Design review of the part built by this model. Coordinates are the model's own, in mm. Coordinates: 2 decimals unless noted, no trailing zeros. Loops run counter-clockwise (first coordinate to the right, second up) from the corner with the lowest first, then second, coordinate; pieces in that order, holes last. Notation, with made-up numbers: M 88,12 L 100,12 A17 cw 100,24 Z; hole C 52.5,3.25 d4. An arc over 180 degrees is marked long. Answer as a JSON object with one key per item and string values. Group by question number.
1. To check wall thickness, follow probe 1 along Z at (x, y) = (76, 8.25); probe 2 along Z at (x, y) = (161, 16.25); probe 3 along Y at (x, z) = (13, -10). State the ranges of each line that lie inside material, in increasing order.
2. Consider section B-B (z = -13). State the section outline as (x, y) points (1 decimal), then the cut area to 3 significant figures.
3. Consider section C-C (x = 68). State the section outline as (y, z) points, then the cut area to 3 significant figures.
4. Consider section A-A (y = 3.75). State the section outline as (x, z) points (3 decimals), then the cut area to 3 significant figures.
5. Insertion check: pin 1 (1 mm diameter, centred on x = 39.5, z = -29.5, fed in from -Y); pin 2 (1 mm diameter, centred on x = 34, y = 17, fed in from -Z); pin 3 (11.5 mm diameter, centred on y = 6, z = -10, fed in from -X). Each pin has a flat end and moves straight along its axis. Give the tip position at first contact, or say it passes through.
6. Consider section D-D (y = 13). State the section outline as (x, z) points.
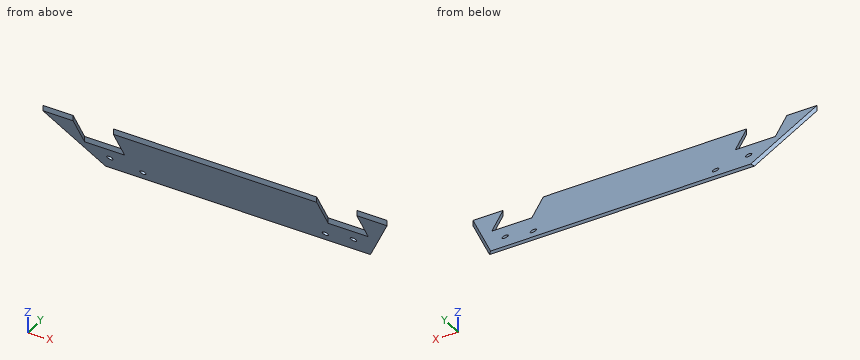
Autodesk Inventor part; units mm, degrees
ref_plane "YZ Plane" through (0, 0, 0) normal (1, 0, 0) x (0, 1, 0)
ref_plane "XZ Plane" through (0, 0, 0) normal (0, 1, 0) x (-1, 0, 0)
ref_plane "XY Plane" through (0, 0, 0) normal (0, 0, 1) x (1, 0, 0)
sketch "Szkic1" plane through (0, 0, 0) normal (1, 0, 0) x (0, 1, 0)
  line L0 (0.433, -0.75) -> (22.433, -38.8551)
  line L1 (22.433, -38.8551) -> (21.134, -39.6051)
  line L2 (21.134, -39.6051) -> (0.433, -3.75)
  line L3 (0.433, -3.75) -> (0.433, -0.75)
  line L4 (21.134, -39.6051) -> (21.134, -39.6051)
  dimension "d0" = 1.5
  dimension "d1" = 22
  dimension "d2" = 30
extrude "Wyciągnięcie proste1" add sketch "Szkic1" along normal blind 180.175
sketch "Szkic2" plane through (180.175, 22.433, 0) normal (0, 0, -1) x (-1, 0, 0)
  line L0 (143.375, -22) -> (164.375, -22)
  line L1 (164.375, -22) -> (164.375, -11.7)
  line L2 (164.375, -11.7) -> (143.375, -11.7)
  line L3 (143.375, -11.7) -> (143.375, -22)
  line L4 (180.175, -22) -> (0, -22) construction
  line L5 (180.175, -22) -> (180.175, 0) construction
  line L6 (180.175, -22) -> (180.175, 0)
  line L7 (180.175, 0) -> (0, 0) construction
  line L8 (158.175, 0) -> (180.175, -22)
  line L9 (90.0875, -22) -> (90.0875, 0) construction
  line L10 (180.175, 0) -> (158.175, 0)
  line L11 (36.8, -22) -> (15.8, -22)
  line L12 (15.8, -22) -> (15.8, -11.7)
  line L13 (15.8, -11.7) -> (36.8, -11.7)
  line L14 (36.8, -11.7) -> (36.8, -22)
  line L15 (0, -22) -> (0, 0) construction
  line L16 (0, -22) -> (0, 0)
  line L17 (22, 0) -> (0, -22)
  line L18 (0, 0) -> (22, 0)
  dimension "d9" = 21
  dimension "d10" = 10.3
  dimension "d33" = 15.8
  dimension "d34" = 45
extrude "Wyciągnięcie proste2" cut sketch "Szkic2" along normal through all
sketch "Szkic3" plane through (22, 22, -38.1051) normal (0, 0.866, 0.5) x (1, 0, 0)
  line L0 (-2, -0.5359) -> (138.175, -0.5359) construction
  line L1 (-2, -0.5359) -> (4.3275, -0.5359) construction
  line L2 (4.3275, -0.5359) -> (4.3275, -10.5359) construction
  line L3 (-2, -0.5359) -> (20.3275, -0.5359) construction
  line L4 (20.3275, -0.5359) -> (20.3275, -6.1359) construction
  line L5 (0, 0.4641) -> (136.175, 0.4641) construction
  line L6 (68.0875, 0.4641) -> (68.0854, -43.134) construction
  line L7 (-22, -43.134) -> (158.175, -43.134) construction
  circle A0 centre (20.3275, -6.1359) radius 1.6
  circle A1 centre (4.3275, -10.5359) radius 1.6
  circle A2 centre (131.8464, -10.542) radius 1.6
  circle A3 centre (115.8469, -6.1405) radius 1.6
  point P0 (-22, -44)
  point P1 (14.8, -43.134)
  point P2 (121.375, -44)
  dimension "d12" = 6.3275
  dimension "d13" = 10
  dimension "d14" = 22.3275
  dimension "d15" = 5.6
  dimension "d16" = 3.2
  dimension "d17" = 3.2
extrude "Wyciągnięcie proste3" cut sketch "Szkic3" against normal through all
properties part number "Przod2mm"
Findings below:
{
 "1": {"probe 1": "z = -17.29 to -14.29", "probe 2": "z = -31.15 to -28.15", "probe 3": "y = 4.04 to 5.77"},
 "2": {"outline": "M 5.3,5.8 L 15.8,5.8 L 15.8,7.5 L 7.1,7.5 Z; M 36.8,5.8 L 143.4,5.8 L 143.4,7.5 L 36.8,7.5 Z; M 164.4,5.8 L 174.8,5.8 L 173.1,7.5 L 164.4,7.5 Z", "area": "218 mm^2"},
 "3": {"outline": "M 0.43,-3.75 L 21.13,-39.61 L 22.43,-38.86 L 0.43,-0.75 Z", "area": "64.1 mm^2"},
 "4": {"outline": "M 3.317,-9.495 L 15.8,-9.495 L 15.8,-6.495 L 3.317,-6.495 Z; M 36.8,-9.495 L 143.375,-9.495 L 143.375,-6.495 L 36.8,-6.495 Z; M 164.375,-9.495 L 176.858,-9.495 L 176.858,-6.495 L 164.375,-6.495 Z", "area": "395 mm^2"},
 "5": {"pin 1": "stops at y = 15.01", "pin 2": "stops at z = -33.31", "pin 3": "stops at x = 1.35"},
 "6": {"outline": "M 12.57,-25.52 L 167.61,-25.52 L 167.61,-22.52 L 12.57,-22.52 Z"}
}
